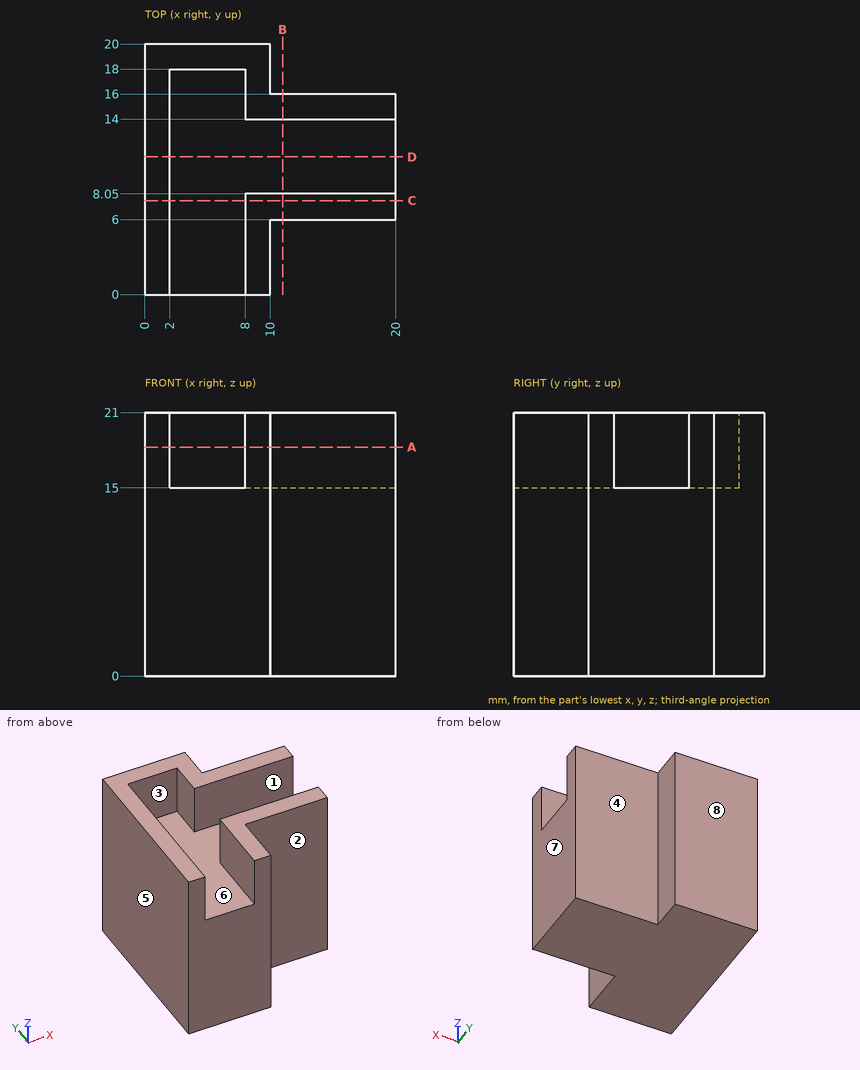
Design review of the part shown in the three views and the two pictorial views. Dimensions are in mm from the part's minimum x, y and z. A direction names the side the tool comes from. Round coordinates to 2 decimals unless told otherwise and drop trailing zeros. Loops run counter-clockwise (first coordinate to the right, second up) from the corner with the lowest first, then second, coordinate; pieces in that order, holes last. Notation, with made-up numbers: (70, -18.5) - (112, -18.5) arc R20 ccw to (112, 20.5) - close; hole circle Ø11 at (71.5, -23.75). An arc over 180 degrees is marked (long way). Write each question's results on one line, items separated by ' | '. Start each with the question number.
Q1. Take a section at B-B on x = 11. Give the boundary of the cut face in (y, z).
Q2. Take a section at D-D on y = 11. Give the boundary of the cut face in (x, z), plus the area to 3 significant figures.
Q3. Draft analysis for pull direction X (two halves, no side actions). For the marked faces 5, 6, 7 and 8, state which applies: pulls with the +X half, pulls with the -X half, needs draft (parallel to the pull), parting line crosses it, or undercut.
Q4. Tool access review of the marked faces 1, 2, 3 and 4: name each direction out of +Z, -Z, +X, -X, +Y, -Y from which nothing blocks a thin tool from reaching the whole face with its end or side.
Q5. Insertion check: P1, Ø5, axis at x = 15.5, z = 6, coming from the +Y side; P2, Ø8, axis at x = 16.5, z = 12, coming from the -Y side; P3, Ø3, axis at y = 4, z = 7, coming from the +X side. Each pin has a flat end and moves straight along its axis. Give the tip position at first contact, or say it passes through.
Q6. Take a section at C-C on y = 7.5. Give the boundary of the cut face in (x, z), plus the area to 3 significant figures.
Q7. Wall thickness on line 1 along Y through (x, z) = (18.5, 18.25); line 2 along X through (y, z) = (1.75, 19); line 3 along X through (y, z) = (15.25, 17): over which ranges is each line inside the solid? List them lowest first. Write a range as [from, to].
Q8. Take a section at A-A on z = 18.25. Give the boundary of the cut face in (x, y).
Data:
1) outline: (6, 0) - (16, 0) - (16, 21) - (14, 21) - (14, 15) - (8.05, 15) - (8.05, 21) - (6, 21) - close
2) outline: (0, 0) - (20, 0) - (20, 15) - (2, 15) - (2, 21) - (0, 21) - close | area: 312 mm²
3) face 5: pulls with the -X half | face 6: undercut | face 7: pulls with the +X half | face 8: needs draft
4) face 1: +Z, +X | face 2: +Z, -Z, +X, -Y | face 3: +Z, -Y | face 4: +Z, -Z, +X, +Y
5) P1: stops at y = 16 | P2: stops at y = 6 | P3: stops at x = 10
6) outline: (0, 0) - (20, 0) - (20, 21) - (8, 21) - (8, 15) - (2, 15) - (2, 21) - (0, 21) - close | area: 384 mm²
7) line 1: y = [6, 8.05], [14, 16] | line 2: x = [0, 2], [8, 10] | line 3: x = [0, 2], [8, 20]
8) outline: (0, 0) - (2, 0) - (2, 18) - (8, 18) - (8, 14) - (20, 14) - (20, 16) - (10, 16) - (10, 20) - (0, 20) - close; (8, 0) - (10, 0) - (10, 6) - (20, 6) - (20, 8.05) - (8, 8.05) - close
